from build123d import *

# Parameters (mm, degrees)
PAD_DEPTH          = 4
POLARPATTERN_COUNT = 3
SKETCH002_R        = 5.4
PAD001_DEPTH       = 22
POCKET_DEPTH       = 14.8
POCKET001_DEPTH    = 0.2
POCKET002_DEPTH    = 26.001
CHAMFER_SIZE       = 0.9
CHAMFER001_SIZE    = 0.9


with BuildPart() as part:
    # Sketch → Pad (new body)
    with BuildSketch(Plane.XY):
        with BuildLine():
            Line((14, 1), (14, -1))
            ThreePointArc((13, -2), (13.707107, -1.707107), (14, -1))
            Line((13, -2), (10.392305, -2))
            ThreePointArc((10.392305, -2), (8.392305, -2.535898), (6.928203, -4))
            ThreePointArc((6.928203, 4), (-8, 0), (6.928203, -4))
            ThreePointArc((6.928203, 4), (8.392305, 2.535898), (10.392305, 2))
            Line((13, 2), (10.392305, 2))
            ThreePointArc((14, 1), (13.707107, 1.707107), (13, 2))
        make_face()
    pad = extrude(amount=PAD_DEPTH)

    # PolarPattern: Pad ×3 about axis
    polarpattern_axis = Axis((0, 0, 0), (0, 0, 1))
    for i in range(1, POLARPATTERN_COUNT):
        add(pad.rotate(polarpattern_axis, i * 360 / POLARPATTERN_COUNT))

    # Sketch002 → Pad001 (join)
    with BuildSketch(Plane.XY.offset(4)):
        Circle(SKETCH002_R)
    extrude(amount=PAD001_DEPTH)

    # Sketch001 → Pocket (cut)
    with BuildSketch(Plane.XY):
        with BuildLine():
            ThreePointArc((-1, 4.2), (-5.2, 0), (-1, -4.2))
            Line((-1, -4.2), (1, -4.2))
            ThreePointArc((1, -4.2), (5.2, 0), (1, 4.2))
            Line((-1, 4.2), (1, 4.2))
        make_face()
    extrude(amount=POCKET_DEPTH, mode=Mode.SUBTRACT)

    # Sketch005 → Pocket001 (cut)
    with BuildSketch(Plane.XY.offset(15)):
        Polygon((-1, 4.2), (-4.614425, 2.139143), (-4.614425, -2.139143), (-1, -4.2), (1, -4.2), (4.614425, -2.139143), (4.614425, 2.139143), (1, 4.2), align=None)
    extrude(amount=-POCKET001_DEPTH, mode=Mode.SUBTRACT)

    # Sketch004 → Pocket002 (cut, through all)
    with BuildSketch(Plane.XY):
        Polygon((4.156922, -2.4), (4.156922, 2.4), (0, 4.8), (-4.156922, 2.4), (-4.156922, -2.4), (0, -4.8), align=None)
    extrude(amount=POCKET002_DEPTH, mode=Mode.SUBTRACT)

    # Chamfer
    chamfer_edges = [part.edges().sort_by_distance(p)[0] for p in [
        (13.707107, 1.707107, 4),
        (14, 0, 4),
        (11.696152, 2, 4),
        (13.707107, -1.707107, 4),
        (8.392305, 2.535898, 4),
        (11.696152, -2, 4),
        (4, 6.928203, 4),
        (8.392305, -2.535898, 4),
        (-2, 8.535898, 4),
        (4, -6.928203, 4),
        (-4.116025, 11.129165, 4),
        (-2, -8.535898, 4),
        (-5.375156, 12.724256, 4),
        (-4.116025, -11.129165, 4),
        (-7, 12.124356, 4),
        (-5.375156, -12.724256, 4),
        (-8.331951, 11.017149, 4),
        (-7, -12.124356, 4),
        (-7.580127, 9.129165, 4),
        (-8.331951, -11.017149, 4),
        (-6.392305, 6, 4),
        (-7.580127, -9.129165, 4),
        (-8, 0, 4),
        (-6.392305, -6, 4),
        (-5.4, 0, 4),
    ]]
    chamfer(chamfer_edges, length=CHAMFER_SIZE)

    # Chamfer001
    chamfer001_edges = [part.edges().sort_by_distance(p)[0] for p in [
        (13.707107, 1.707107, 0),
        (14, 0, 0),
        (11.696152, 2, 0),
        (13.707107, -1.707107, 0),
        (8.392305, 2.535898, 0),
        (11.696152, -2, 0),
        (4, 6.928203, 0),
        (8.392305, -2.535898, 0),
        (-2, 8.535898, 0),
        (4, -6.928203, 0),
        (-4.116025, 11.129165, 0),
        (-2, -8.535898, 0),
        (-5.375156, 12.724256, 0),
        (-4.116025, -11.129165, 0),
        (-7, 12.124356, 0),
        (-5.375156, -12.724256, 0),
        (-8.331951, 11.017149, 0),
        (-7, -12.124356, 0),
        (-7.580127, 9.129165, 0),
        (-8.331951, -11.017149, 0),
        (-6.392305, 6, 0),
        (-7.580127, -9.129165, 0),
        (-8, 0, 0),
        (-6.392305, -6, 0),
        (-0.519777, 4.499907, 0),
        (0.519777, 4.499907, 0),
        (5.2, 0, 0),
        (0.519777, -4.499907, 0),
        (-0.519777, -4.499907, 0),
        (-5.2, 0, 0),
    ]]
    chamfer(chamfer001_edges, length=CHAMFER001_SIZE)


solid = part.part
Can you work these out from the model? Positions are in its coordinate system, mm. A direction names the side the tool comes from. Coordinates: 2 decimals unless noted, no trailing zeros. Order: outer loops, then holes, each group sorted by start corner. A loop starts at its lowest first (then second) coordinate and runs counter-clockwise, first axis right, second up. Notation, with made-up numbers: M 61,12.25 L 68,12.25 A24 ccw 68,38.25 Z; hole C 86.25,-0.75 d4. An arc over 180 degrees is marked long. Answer as CSV lines item,"result".
(1) On a 3-axis mill with a long thin cutter (end or side, diameter ignored), from which of +Z, -Z, +X, -X, +Y, -Y can I reach the whole of each face in a straight line? I mean faces 4 (the flat face through (3, -3.4, 14.8)), 5 (the flat face through (1.59, -3.88, 18.85)), 6 (the flat face through (-7.589, -9.145, 1.985)), 7 (the flat face through (11.7, 1.6, 0.5)). Say none if no direction works.
Geometry check:
face 4,"-Z"
face 5,"+Z, -Z"
face 6,"+Z, -Z, -X"
face 7,"-Z, +X, +Y"
(2) Suppose I cut it at C-C on z = 11.75. Please give me the cut outline in (x, y), plus the area to 3 significant figures.
Geometry check:
outline,"C 0,0 d10.8; hole M -1.04,-4.2 L 0,-4.8 L 1.04,-4.2 A4.2 ccw 1.04,4.2 L 0,4.8 L -1.04,4.2 A4.2 ccw Z"
area,"18.1 mm^2"
(3) I'm going to push flat-ended pins straight in: pin 1 (2 mm diameter, centred on y = -5, z = 4, fed in from +X); pin 2 (1.1 mm diameter, centred on x = 12, z = 2, fed in from -Y); pin 3 (1.5 mm diameter, centred on y = -2.5, z = 11, fed in from +X); pin 4 (1 mm diameter, centred on x = -2, y = 3, fed in from -Z). Where does each tip first touch, or does it pass through?
Geometry check:
pin 1,"x = 6.57"
pin 2,"y = -2"
pin 3,"x = 5.11"
pin 4,"through"
(4) Please list where these lines run through material, in increasing order: L1, parallel to Z at x = -3.5, y = 8; L2, parallel to X at y = 1.25, z = 24.5; L3, parallel to Y at x = 2.25, z = 18.25.
Geometry check:
L1,"0 to 4"
L2,"-5.25 to -4.16, 4.16 to 5.25"
L3,"-4.91 to -3.5, 3.5 to 4.91"
(5) If we mould it in two halves opening along X, with no side actions, what happens to faces 1 (the flat face through (-0.506, 5.02, 0.456)), 2 (the cylindrical face through (8.37, 2.55, 1.98)), 3 (the cylindrical face through (-6.392, -6.029, 1.985))? For each: released by +X, released by -X, zero draft, split by the parting line, or undercut.
Geometry check:
face 1,"undercut"
face 2,"released by +X"
face 3,"released by -X"
(6) Suppose I cut it at B-B on x = 11.25. Please give me the cut outline in (y, z), plus the area to 3 significant figures.
Geometry check:
outline,"M -2,0.9 L -1.1,0 L 1.1,0 L 2,0.9 L 2,3.1 L 1.1,4 L -1.1,4 L -2,3.1 Z"
area,"14.4 mm^2"
